```python
from build123d import *

# Parameters (mm, degrees)
SZKIC1_W                    = 54
SZKIC1_H                    = 71
DODANIE_WYCI_GNI_CIE1_DEPTH = 5
SZKIC2_W                    = 23.5
SZKIC2_H                    = 28
WYTNIJ_WYCI_GNI_CIE1_DEPTH  = 5
SZKIC3_W                    = 21
SZKIC3_H                    = 21
WYTNIJ_WYCI_GNI_CIE2_DEPTH  = 3
SZKIC4_R                    = 1.5
WYTNIJ_WYCI_GNI_CIE3_DEPTH  = 5
SZKIC5_W                    = 20
SZKIC5_H                    = 43
DODANIE_WYCI_GNI_CIE2_DEPTH = 5
SZKIC6_R                    = 8.5
WYTNIJ_WYCI_GNI_CIE4_DEPTH  = 5
SZKIC7_R                    = 3
WYTNIJ_WYCI_GNI_CIE5_DEPTH  = 10
ZAOKR_GLENIE3_R             = 10
SZKIC8_W                    = 19
SZKIC8_H                    = 28
DODANIE_WYCI_GNI_CIE3_DEPTH = 5
ZAOKR_GLENIE2_SIZE          = 2
SZKIC9_R                    = 2
WYTNIJ_WYCI_GNI_CIE6_DEPTH  = 10
SFAZOWANIE2_SIZE            = 1
SFAZOWANIE3_SIZE            = 0.5
SZKIC10_R                   = 1.5
WYTNIJ_WYCI_GNI_CIE7_DEPTH  = 10


with BuildPart() as part:
    # Szkic1 → Dodanie-wyciągnięcie1 (new body)
    with BuildSketch(Plane.XY):
        with Locations((7, 0.5)):
            Rectangle(SZKIC1_W, SZKIC1_H)
    extrude(amount=DODANIE_WYCI_GNI_CIE1_DEPTH)

    # Szkic2 → Wytnij-wyciągnięcie1 (cut)
    with BuildSketch(Plane.XY.offset(5)):
        with Locations((-8.25, 22)):
            Rectangle(SZKIC2_W, SZKIC2_H)
    extrude(amount=-WYTNIJ_WYCI_GNI_CIE1_DEPTH, mode=Mode.SUBTRACT)

    # Szkic3 → Wytnij-wyciągnięcie2 (cut)
    with BuildSketch(Plane(origin=(0, 0, 0), x_dir=(-1, 0, 0), z_dir=(0, 0, -1))):
        with Locations((-14, 20)):
            Rectangle(SZKIC3_W, SZKIC3_H)
    extrude(amount=-WYTNIJ_WYCI_GNI_CIE2_DEPTH, mode=Mode.SUBTRACT)

    # Szkic4 → Wytnij-wyciągnięcie3 (cut)
    with BuildSketch(Plane.XY.offset(5)):
        with Locations((6, 32.5)):
            Circle(SZKIC4_R)
        with Locations((14, 32.5)):
            Circle(SZKIC4_R)
        with Locations((22, 32.5)):
            Circle(SZKIC4_R)
        with Locations((22, 5.5)):
            Circle(SZKIC4_R)
        with Locations((6, 5.5)):
            Circle(SZKIC4_R)
        with Locations((27.5, 27)):
            Circle(SZKIC4_R)
        with Locations((27.5, 11)):
            Circle(SZKIC4_R)
    extrude(amount=-WYTNIJ_WYCI_GNI_CIE3_DEPTH, mode=Mode.SUBTRACT)

    # Szkic5 → Dodanie-wyciągnięcie2 (add)
    with BuildSketch(Plane.XY.offset(5)):
        with Locations((-30, -13.5)):
            Rectangle(SZKIC5_W, SZKIC5_H)
    extrude(amount=-DODANIE_WYCI_GNI_CIE2_DEPTH)

    # Szkic6 → Wytnij-wyciągnięcie4 (cut)
    with BuildSketch(Plane.XY.offset(5)):
        with Locations((-20, -4)):
            Circle(SZKIC6_R)
        with Locations((14, -4)):
            Circle(SZKIC6_R)
    extrude(amount=-WYTNIJ_WYCI_GNI_CIE4_DEPTH, mode=Mode.SUBTRACT)

    # Szkic7 → Wytnij-wyciągnięcie5 (cut)
    with BuildSketch(Plane.XY.offset(5)):
        with Locations((-11, -30)):
            Circle(SZKIC7_R)
        with Locations((5, -30)):
            Circle(SZKIC7_R)
        with Locations((-35, -19)):
            Circle(SZKIC7_R)
        with Locations((29, -19)):
            Circle(SZKIC7_R)
    extrude(amount=-WYTNIJ_WYCI_GNI_CIE5_DEPTH, mode=Mode.SUBTRACT)

    # Zaokrąglenie3
    zaokr_glenie3_edges = [part.edges().sort_by_distance(p)[0] for p in [
        (-40, -35, 2.5),
        (34, -35, 2.5),
    ]]
    fillet(zaokr_glenie3_edges, radius=ZAOKR_GLENIE3_R)

    # Szkic8 → Dodanie-wyciągnięcie3 (add)
    with BuildSketch(Plane.XY.offset(5)):
        with Locations((-30.5, 22)):
            Rectangle(SZKIC8_W, SZKIC8_H)
    extrude(amount=-DODANIE_WYCI_GNI_CIE3_DEPTH)

    # Zaokrąglenie2
    # a fillet whose section is not a circle: 2 mm, written as the material it adds along each edge
    with BuildSketch(Plane(origin=(3.5, 8, 5), x_dir=(0, 1, 0), z_dir=(0, 0, -1))) as zaokr_glenie2_piece_1_section:
        with BuildLine():
            Bezier((ZAOKR_GLENIE2_SIZE, 0), (0, 0), (0, -ZAOKR_GLENIE2_SIZE), weights=[1, 1, 1])
            Line((0, -ZAOKR_GLENIE2_SIZE), (0, 0))
            Line((0, 0), (ZAOKR_GLENIE2_SIZE, 0))
        make_face()
    zaokr_glenie2_piece_1 = extrude(amount=5, mode=Mode.PRIVATE)
    zaokr_glenie2_piece_1 = split(zaokr_glenie2_piece_1, bisect_by=Plane(origin=(3.5, 9.5, 5), z_dir=(0, 1, 0)), keep=Keep.TOP, mode=Mode.PRIVATE)
    zaokr_glenie2_piece_1 = split(zaokr_glenie2_piece_1, bisect_by=Plane(origin=(3.5, 8, 3), z_dir=(0, 0, 1)), keep=Keep.TOP, mode=Mode.PRIVATE)
    add(zaokr_glenie2_piece_1)
    with BuildSketch(Plane(origin=(3.5, 8, 5), x_dir=(0, 1, 0), z_dir=(0, 0, -1))) as zaokr_glenie2_piece_2_section:
        with BuildLine():
            Bezier((ZAOKR_GLENIE2_SIZE, 0), (0, 0), (0, -ZAOKR_GLENIE2_SIZE), weights=[1, 1, 1])
            Line((0, -ZAOKR_GLENIE2_SIZE), (0, 0))
            Line((0, 0), (ZAOKR_GLENIE2_SIZE, 0))
        make_face()
    zaokr_glenie2_piece_2 = extrude(amount=5, mode=Mode.PRIVATE)
    zaokr_glenie2_piece_2 = split(zaokr_glenie2_piece_2, bisect_by=Plane(origin=(3.5, 9.5, 5), z_dir=(0, -1, 0)), keep=Keep.TOP, mode=Mode.PRIVATE)
    zaokr_glenie2_piece_2 = split(zaokr_glenie2_piece_2, bisect_by=Plane(origin=(3.5, 8, 3), z_dir=(0, 0, 1)), keep=Keep.TOP, mode=Mode.PRIVATE)
    add(zaokr_glenie2_piece_2)
    with BuildSketch(Plane(origin=(3.5, 8, 5), x_dir=(0, 1, 0), z_dir=(0, 0, -1))) as zaokr_glenie2_piece_3_section:
        with BuildLine():
            Bezier((ZAOKR_GLENIE2_SIZE, 0), (0, 0), (0, -ZAOKR_GLENIE2_SIZE), weights=[1, 1, 1])
            Line((0, -ZAOKR_GLENIE2_SIZE), (0, 0))
            Line((0, 0), (ZAOKR_GLENIE2_SIZE, 0))
        make_face()
    zaokr_glenie2_piece_3 = extrude(amount=5, mode=Mode.PRIVATE)
    zaokr_glenie2_piece_3 = split(zaokr_glenie2_piece_3, bisect_by=Plane(origin=(3.5, 9.5, 5), z_dir=(0, -1, 0)), keep=Keep.TOP, mode=Mode.PRIVATE)
    zaokr_glenie2_piece_3 = split(zaokr_glenie2_piece_3, bisect_by=Plane(origin=(3.5, 8, 3), z_dir=(0, 0, -1)), keep=Keep.TOP, mode=Mode.PRIVATE)
    add(zaokr_glenie2_piece_3)
    with BuildSketch(Plane(origin=(-21, 8, 5), x_dir=(1, 0, 0), z_dir=(0, 0, -1))) as zaokr_glenie2_piece_4:
        with BuildLine():
            Bezier((ZAOKR_GLENIE2_SIZE, 0), (0, 0), (0, -ZAOKR_GLENIE2_SIZE), weights=[1, 1, 1])
            Line((0, -ZAOKR_GLENIE2_SIZE), (0, 0))
            Line((0, 0), (ZAOKR_GLENIE2_SIZE, 0))
        make_face()
    extrude(amount=5)

    # Szkic9 → Wytnij-wyciągnięcie6 (cut)
    with BuildSketch(Plane.XY.offset(5)):
        with Locations((-27, 31)):
            Circle(SZKIC9_R)
        with Locations((-27, 21)):
            Circle(SZKIC9_R)
    extrude(amount=-WYTNIJ_WYCI_GNI_CIE6_DEPTH, mode=Mode.SUBTRACT)

    # Sfazowanie2
    sfazowanie2_edges = [part.edges().sort_by_distance(p)[0] for p in [
        (-30.5, 36, 0),
        (-30.5, 36, 5),
        (18.75, 36, 5),
        (18.75, 36, 0),
    ]]
    chamfer(sfazowanie2_edges, length=SFAZOWANIE2_SIZE)

    # Sfazowanie3
    sfazowanie3_edges = [part.edges().sort_by_distance(p)[0] for p in [
        (-28.5, -4, 5),
        (5.5, -4, 5),
    ]]
    chamfer(sfazowanie3_edges, length=SFAZOWANIE3_SIZE)

    # Szkic10 → Wytnij-wyciągnięcie7 (cut)
    with BuildSketch(Plane.XY.offset(5)):
        with Locations((-3, -21)):
            Circle(SZKIC10_R)
    extrude(amount=-WYTNIJ_WYCI_GNI_CIE7_DEPTH, mode=Mode.SUBTRACT)


solid = part.part
```
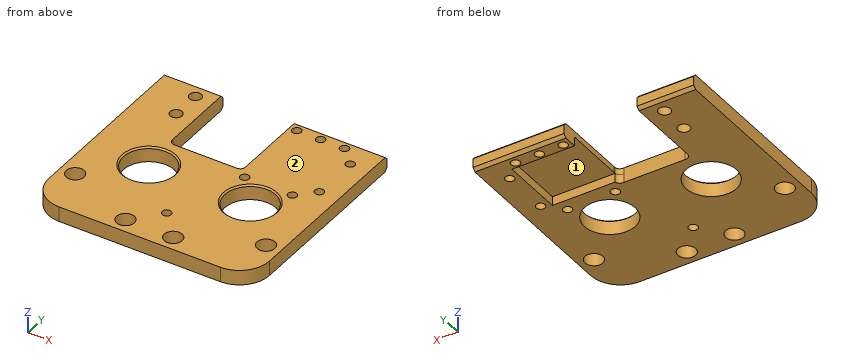
Model file for the job. Use its own axes, mm. Face numbers are marked on the shaded views. Coordinates: 2 decimals unless noted, no trailing zeros. Write each loop counter-clockwise with the first axis right and the second up, starting at its lowest first coordinate (ties: lowest second). Pieces come first, ordered by that corner, then holes. Notation, with made-up numbers: (80, 25.25) - (94, 25.25) arc R23 cw to (94, 39.25) - close; hole circle Ø7 at (83.25, -16). An arc over 180 degrees is marked (long way). One line per item, written item: value. Start each with the question number.
1. Slice it at B-B (x = -33). Write the cut outline in (y, z).
2. Mould opens along Y. For the marked faces 1 and 2 say: released by +Y, released by -Y, zero draft, split by the parting line, or undercut.
3. Probe line 1 (Y direction, x = 14, z = 1.9); line 2 (Y direction, x = 18, z = 2.4); line 3 (Y direction, x = 14, z = 3.6). List the from-to ranges inside material, lowest first. Write a range as from..to.
4. Slice it at A-A (y = 27). Write the cut outline in (x, z).
5. Flat gauge pin, fed straight in: pin 1 (2.5 mm diameter, centred on x = -3, y = -21, fed in from +Z). Where does the tip first touch, or does it go through?
6. Slice it at C-C (z = 2). Count the separate pieces of the cut face and the enclosed holes in it, plus the area to 3 significant figures.
Answers below:
1. outline: (-34.54, 0) - (-21.24, 0) - (-21.24, 5) - (-34.54, 5) - close; (-16.76, 0) - (35, 0) - (36, 1) - (36, 4) - (35, 5) - (-16.76, 5) - close
2. face 1: undercut
2. face 2: zero draft
3. line 1: y = -35..-12.5, 4.5..9.5, 30.5..31, 34..36
3. line 2: y = -35..-11.5, 3.5..9.5, 30.5..36
3. line 3: y = -35..-12.5, 4.5..31, 34..36
4. outline: (-40, 0) - (-21, 0) - (-21, 5) - (-40, 5) - close; (3.5, 3) - (24.5, 3) - (24.5, 0) - (26, 0) - (26, 5) - (3.5, 5) - close; (29, 0) - (34, 0) - (34, 5) - (29, 5) - close
5. pin 1: passes through
6. separate pieces: 1
6. enclosed holes: 16
6. area: 3,440 mm^2
